from build123d import *

# Parameters (mm, degrees)
BOX002_W                    = 20
BOX002_H                    = 2.5
BOX002_DEPTH                = 8
BOX_W                       = 5
BOX_H                       = 20
BOX_DEPTH                   = 5
BOX001_W                    = 20
BOX001_H                    = 7
BOX001_DEPTH                = 10
CYLINDER001_W               = 52
CYLINDER001_H               = 15
CYLINDER001_ANGLE           = 60
CYLINDER001_PLACEMENT_ANGLE = 60
CYLINDER_W                  = 54
CYLINDER_H                  = 15
CYLINDER_ANGLE              = 60
CYLINDER_PLACEMENT_ANGLE    = 60


with BuildPart() as slot:
    # Box002 → Box002 (new body)
    with BuildSketch(Plane(origin=(3, 46, 3.5), x_dir=(1, 0, 0), z_dir=(0, 0, 1))):
        with Locations((10, 1.25)):
            Rectangle(BOX002_W, BOX002_H)
    extrude(amount=BOX002_DEPTH)


with BuildPart() as pin_opening:
    # Box → Box (new body)
    with BuildSketch(Plane(origin=(7, 42, 5), x_dir=(1, 0, 0), z_dir=(0, 0, 1))):
        with Locations((2.5, 10)):
            Rectangle(BOX_W, BOX_H)
    extrude(amount=BOX_DEPTH)


with BuildPart() as latch:
    # Box001 → Box001 (new body)
    with BuildSketch(Plane(origin=(0, 44, 2.5), x_dir=(1, 0, 0), z_dir=(0, 0, 1))):
        with Locations((10, 3.5)):
            Rectangle(BOX001_W, BOX001_H)
    extrude(amount=BOX001_DEPTH)


with BuildPart() as bottle_wall001:
    # Cylinder001 → Cylinder001 (revolve)
    with BuildSketch(Plane.XZ):
        with Locations((26, 7.5)):
            Rectangle(CYLINDER001_W, CYLINDER001_H)
    revolve(axis=Axis((0, 0, 0), (0, 0, 1)), revolution_arc=CYLINDER001_ANGLE)


with BuildPart() as bottle_wall001_1:
    # Cylinder001 placement: moved
    add(bottle_wall001.part.moved(Location((8.5, -7, 0))).rotate(Axis((8.5, -7, 0), (0, 0, 1)), CYLINDER001_PLACEMENT_ANGLE))


with BuildPart() as cut002:
    # Cylinder → Cylinder (revolve)
    with BuildSketch(Plane.XZ):
        with Locations((27, 7.5)):
            Rectangle(CYLINDER_W, CYLINDER_H)
    revolve(axis=Axis((0, 0, 0), (0, 0, 1)), revolution_arc=CYLINDER_ANGLE)


with BuildPart() as cut002_1:
    # Cylinder placement: moved
    add(cut002.part.moved(Location((8.5, -7, 0))).rotate(Axis((8.5, -7, 0), (0, 0, 1)), CYLINDER_PLACEMENT_ANGLE))

    # Cut: cut bottle_wall001
    add(bottle_wall001_1.part, mode=Mode.SUBTRACT)


with BuildPart() as cut002_2:
    # Cut placement: moved
    add(cut002_1.part.moved(Location((0, -2, 0))))

    # Fusion: union latch
    add(latch.part)

    # Fusion001: union latch
    add(latch.part)

    # Cut001: cut pin_opening
    add(pin_opening.part, mode=Mode.SUBTRACT)

    # Cut002: cut slot
    add(slot.part, mode=Mode.SUBTRACT)


solid = cut002_2.part
Check sheet for the modelled part. Datum: model origin and axes. Units: mm. A direction names the side the tool comes from. Give positions to 0.01 mm unless a question says otherwise; leave off trailing zeros. Loops run counter-clockwise (first coordinate to the right, second up) from the corner with the lowest first, then second, coordinate; pieces in that order, holes last. Notation, with made-up numbers: M -24.75,85 L -6.75,85 A9 cw -6.75,100 Z; hole C -7,-14.75 d7. An arc over 180 degrees is marked long. Return JSON: item names as keys, results as strings. Group by question number.
1. Cross-section at C-C on z = 4.5. Record the boundary of the cut face in (x, y).
2. Cross-section at B-B on x = 11. Record the boundary of the cut face in (y, z).
3. Go/stop test with flat-tipped pins: pin 1 (1.6 mm diameter, centred on x = 8.5, y = 44.5, fed in from -Z); pin 2 (0.8 mm diameter, centred on y = 50.5, z = 6.5, fed in from +X); pin 3 (0.8 mm diameter, centred on y = 47.5, z = 7, fed in from +X); pin 4 (3 mm diameter, centred on y = 50, z = 8.5, fed in from -X). Record where each tip stops, or that it passes through.
4. Cross-section at A-A on z = 9.5. Record the boundary of the cut face in (x, y), plus the area to 3 significant figures.
5. Thickness scan on L1, parallel to Z at x = 6.5, y = 46.75; L2, parallel to X at y = 46.5, z = 6; L3, parallel to X at y = 39, z = 3. Record the ranges inside material, lowest first.
6. Mould release check, pull along Z, two halves, no side actions. Record for faces 5 (the flat face through (3, 47, 7)), 6 (the flat face through (9, 50, 5)), 7 (the flat face through (-18, 36.9, 7.6)), 8 (the flat face through (8, 44, 15)): released by +Z, released by -Z, zero draft, split by the parting line, or undercut.
7. Tool access check on faces 1 (the flat face through (7, 44, 7)), 2 (the flat face through (10, 51, 11)), 3 (the flat face through (13, 48.5, 7)), 4 (the flat face through (0, 48, 7)). Record the directions out of +Z, -Z, +X, -X, +Y, -Y that give a thin tool (end or side, any length) a straight path to the whole face; none if there is none.
8. Cross-section at D-D on y = 49.5. Record the boundary of the cut face in (x, z), plus the area to 3 significant figures.
Return value:
{
 "1": {"outline": "M -18.5,37.77 L -17.5,36.03 A52 cw 34.5,36.03 L 35.5,37.77 A54 ccw 18.84,44 L 20,44 L 20,46 L 3,46 L 3,48.5 L 20,48.5 L 20,51 L 0,51 L 0,44.33 A54 ccw Z"},
 "2": {"outline": "M 42.94,0 L 44.94,0 L 44.94,2.5 L 51,2.5 L 51,5 L 48.5,5 L 48.5,3.5 L 46,3.5 L 46,5 L 42.94,5 Z; M 42.94,10 L 46,10 L 46,11.5 L 48.5,11.5 L 48.5,10 L 51,10 L 51,12.5 L 44.94,12.5 L 44.94,15 L 42.94,15 Z"},
 "3": {"pin 1": "z = 0", "pin 2": "x = 20", "pin 3": "x = 3", "pin 4": "x = 0"},
 "4": {"outline": "M -18.5,37.77 L -17.5,36.03 A52 cw 7,42.98 L 7,46 L 3,46 L 3,48.5 L 7,48.5 L 7,51 L 0,51 L 0,44.33 A54 ccw Z; M 12,42.88 A52 cw 34.5,36.03 L 35.5,37.77 A54 ccw 18.84,44 L 20,44 L 20,46 L 12,46 Z; M 12,48.5 L 20,48.5 L 20,51 L 12,51 Z", "area": "167 mm^2"},
 "5": {"L1": "2.5 to 3.5, 11.5 to 12.5", "L2": "0 to 3", "L3": "-16.24 to -11.5, 28.5 to 33.24"},
 "6": {"face 5": "undercut", "face 6": "undercut", "face 7": "zero draft", "face 8": "released by +Z"},
 "7": {"face 1": "+Y, -Y", "face 2": "+Z, -Z, +X, -X, +Y", "face 3": "+X", "face 4": "+Z, -Z, -X, +Y"},
 "8": {"outline": "M 0,2.5 L 20,2.5 L 20,12.5 L 0,12.5 Z; hole M 7,5 L 12,5 L 12,10 L 7,10 Z", "area": "175 mm^2"}
}
